from build123d import *

# Parameters (mm, degrees)
SALIENTE_EXTRUIR1_DEPTH       = 100
SALIENTE_EXTRUIR2_DEPTH       = 6.35
TALADRO_ROSCADO_1_4_202_D     = 5.1054
TALADRO_ROSCADO_8_321_D       = 3.4544
TALADRO_ROSCADO_8_321_DEPTH   = 4.7625
TALADRO_ROSCADO_8_321_TIP     = 1.037806461
CROQUIS10_R                   = 6.5
CORTAR_EXTRUIR1_DEPTH         = 111.761638779
CORTAR_EXTRUIR2_DEPTH         = 6.35
TALADRO_ROSCADO_1_4_203_D     = 5.1054
TALADRO_ROSCADO_1_4_203_DEPTH = 13
TALADRO_ROSCADO_1_4_203_TIP   = 1.533816902
F_3_8_16_TAPPED_HOLE1_D       = 7.9375
F_3_8_16_TAPPED_HOLE1_DEPTH   = 23.81
F_3_8_16_TAPPED_HOLE1_TIP     = 2.384665582


with BuildPart() as part:
    # Croquis1 → Saliente-Extruir1 (new, symmetric)
    with BuildSketch(Plane.XY):
        Polygon((12.7, 28.575), (0, 28.575), (0, 0), (0, -28.575), (38.1, -28.575), (38.1, -22.225), (12.7, -22.225), (12.7, 22.225), align=None)
    extrude(amount=SALIENTE_EXTRUIR1_DEPTH, both=True)

    # Croquis2 → Saliente-Extruir2 (add, symmetric)
    with BuildSketch(Plane(origin=(0, 0, 0), x_dir=(1, 0, 0), z_dir=(0, 1, 0))):
        Polygon((0, 50), (0, -50), (-19.05, -30.95), (-19.05, 30.95), align=None)
    extrude(amount=SALIENTE_EXTRUIR2_DEPTH, both=True)

    # Taladro roscado 1/4-202 (through all)
    with Locations(Plane.XY.offset(50)):
        with Locations((-9.525, 0)):
            Hole(TALADRO_ROSCADO_1_4_202_D / 2)

    # Taladro roscado #8-321
    with Locations(Plane.ZY.offset(19.05)):
        with Locations((0, 0)):
            Hole(TALADRO_ROSCADO_8_321_D / 2, depth=TALADRO_ROSCADO_8_321_DEPTH)
            with Locations((0, 0, -(TALADRO_ROSCADO_8_321_DEPTH + TALADRO_ROSCADO_8_321_TIP / 2))):  # 118° drill point
                Cone(0, TALADRO_ROSCADO_8_321_D / 2, TALADRO_ROSCADO_8_321_TIP, mode=Mode.SUBTRACT)

    # Croquis10 → Cortar-Extruir1 (cut, through all)
    with BuildSketch(Plane.ZY):
        with Locations(Location((80, 10, 0), (0, 0, 270))):
            Circle(CROQUIS10_R)
    extrude(amount=-CORTAR_EXTRUIR1_DEPTH, mode=Mode.SUBTRACT)

    # Croquis13 → Cortar-Extruir2 (cut)
    with BuildSketch(Plane.XZ.offset(28.575)):
        with BuildLine():
            Line((27.225, -10.795039516), (27.225, -30.790076058))
            ThreePointArc((27.225, -30.790076058), (22.225, -35.790076058), (17.225, -30.790076058))
            Line((17.225, -30.790076058), (17.225, -10.795039516))
            ThreePointArc((17.225, -10.795039516), (22.225, -5.795039516), (27.225, -10.795039516))
        make_face()
    extrude(amount=-CORTAR_EXTRUIR2_DEPTH, mode=Mode.SUBTRACT)

    # Taladro roscado 1/4-203
    with Locations(Plane(origin=(12.7, 0, 0), x_dir=(0, 0, 1), z_dir=(1, 0, 0))):
        with Locations((5, -10)):
            Hole(TALADRO_ROSCADO_1_4_203_D / 2, depth=TALADRO_ROSCADO_1_4_203_DEPTH)
            with Locations((0, 0, -(TALADRO_ROSCADO_1_4_203_DEPTH + TALADRO_ROSCADO_1_4_203_TIP / 2))):  # 118° drill point
                Cone(0, TALADRO_ROSCADO_1_4_203_D / 2, TALADRO_ROSCADO_1_4_203_TIP, mode=Mode.SUBTRACT)

    # 3/8-16 Tapped Hole1
    with Locations(Plane(origin=(0, -28.575, 0), x_dir=(-1, 0, 0), z_dir=(0, -1, 0))):
        with Locations((-22.225, -9.204960484)):
            Hole(F_3_8_16_TAPPED_HOLE1_D / 2, depth=F_3_8_16_TAPPED_HOLE1_DEPTH)
            with Locations((0, 0, -(F_3_8_16_TAPPED_HOLE1_DEPTH + F_3_8_16_TAPPED_HOLE1_TIP / 2))):  # 118° drill point
                Cone(0, F_3_8_16_TAPPED_HOLE1_D / 2, F_3_8_16_TAPPED_HOLE1_TIP, mode=Mode.SUBTRACT)


solid = part.part
Verification items for the finished model (mm, model axes). A direction names the side the tool comes from. Coordinates: 2 decimals unless noted, no trailing zeros. Order: outer loops, then holes, each group sorted by start corner. A loop starts at its lowest first (then second) coordinate and runs counter-clockwise, first axis right, second up.
Item 1: Material ranges on L1, parallel to Z at x = 4, y = 10; L2, parallel to X at y = 0, z = -16; L3, parallel to Y at x = 4, z = 5 (3 decimals), recorded low to high.
Filled in:
L1: z = -100 to 2.45, 7.55 to 73.5, 86.5 to 100
L2: x = -19.05 to -12.08, -6.97 to 12.7
L3: y = -28.575 to 7.447, 12.553 to 28.575
Item 2: Section check B-B, the plane y = 10. Enter the section's corners in (x, z).
Filled in:
outline: (0, -100) - (12.7, -100) - (12.7, 2.45) - (0, 2.45) - close; (0, 7.55) - (12.7, 7.55) - (12.7, 73.5) - (0, 73.5) - close; (0, 86.5) - (12.7, 86.5) - (12.7, 100) - (0, 100) - close
Item 3: Section check A-A, the plane z = 80. Enter the section's corners in (x, y) (3 decimals), then the cut area to 3 significant figures.
Filled in:
outline: (0, -28.575) - (38.1, -28.575) - (38.1, -22.225) - (12.7, -22.225) - (12.7, 3.5) - (0, 3.5) - close; (0, 16.5) - (12.7, 16.5) - (12.7, 28.575) - (0, 28.575) - close
area: 722 mm2
Item 4: Section check C-C, the plane x = 20. Enter the section's corners in (y, z) (3 decimals).
Filled in:
outline: (-28.575, -100) - (-22.225, -100) - (-22.225, -35.268) - (-28.575, -35.268) - close; (-28.575, -6.317) - (-22.225, -6.317) - (-22.225, 5.919) - (-28.575, 5.919) - close; (-28.575, 12.491) - (-22.225, 12.491) - (-22.225, 100) - (-28.575, 100) - close
Item 5: Access from +Z, -Z, +X, -X, +Y, -Y to the whole of each face (thin tool, end or side, straight path). Record for faces 4 (the face through (22.115, -25.444, -5.796)), 5 (the face through (-9, -6.35, -1)), 6 (the face through (-16.635, 1.713, 0.225)), 7 (the face through (6, 28.575, 1)), 8 (the face through (-9, 6.35, -1)).
Filled in:
face 4: +Y, -Y
face 5: +Z, -Z, -X, -Y
face 6: -X
face 7: +Z, -Z, +X, -X, +Y
face 8: +Z, -Z, -X, +Y
Item 6: Release check for a two-part mould opening along Z. For faces 1 (the face through (-13.43, -0.11, 0.28)), 2 (the face through (-9, -3, 41)), 3 (the face through (0, 7, 1)) record: +Z half, -Z half, draft (parallel to the pull), parting line (faces both ways), or undercut.
Filled in:
face 1: undercut
face 2: +Z half
face 3: draft
Item 7: Depth check by flat-ended pin: pin 1 (8 mm diameter, centred on y = 10, z = 5, fed in from +X); pin 2 (15 mm diameter, centred on x = -8, z = -3.5, fed in from +Y); pin 3 (17 mm diameter, centred on y = -4.5, z = 49, fed in from -X); pin 4 (9 mm diameter, centred on x = 22.22, z = 9.2, fed in from -Y) (3 decimals). Enter the tip coordinate at first touch or a pass-through.
Filled in:
pin 1: stops at x = 12.7
pin 2: stops at y = 6.35
pin 3: stops at x = -9.5
pin 4: stops at y = -28.575
Item 8: Section check D-D, the plane x = -2.5. Enter the section's corners in (y, z).
Filled in:
outline: (-6.35, -47.5) - (6.35, -47.5) - (6.35, 47.5) - (-6.35, 47.5) - close
